Could you check a few things on this model? Use its own coordinates, in mm. Give positions to 0.01 mm unless a question says otherwise; leave off trailing zeros.
1. Imagine slicing it at A-A (y = -387). Count the separate pieces of the cut face and the enclosed holes in it, plus the area to 3 significant figures.
2. For P1, Ø4, axis at y = -136, z = 0, coming from the -X side; P2, Ø3, axis at y = -266, z = -0.5, coming from the +X side; P3, Ø4, axis at x = 1.5, y = -77, coming from the +Z side, each with a flat end and sliding along its axis, tell me the tip position at first contact or that it passes through.
3. I need wall thicknesses on line 1 along Z through (x, y) = (10, -334.5); line 2 along X through (y, z) = (-418.5, -9.5); line 3 along Z through (x, y) = (-11.5, -450). Which ranges of each line are inside material? Lowest first, please.
```python
from build123d import *

# Parameters (mm, degrees)
F0_R     = 3
F0_R_2   = 2.5
F1_DEPTH = 510


with BuildPart() as f1:
    # F0 (on Front) → F1 (new body)
    with BuildSketch(Plane.XZ):
        with BuildLine():
            Line((-4.5, 15), (-14, 15))
            ThreePointArc((-14, 15), (-14.707107, 14.707107), (-15, 14))
            Line((-15, 14), (-15, 4.5))
            ThreePointArc((-15, 4.5), (-14.912132, 4.287868), (-14.7, 4.2))
            Line((-14.7, 4.2), (-14.5, 4.2))
            ThreePointArc((-14.5, 4.2), (-14.146447, 4.053553), (-14, 3.7))
            Line((-14, 3.7), (-14, 3.55))
            ThreePointArc((-14, 3.55), (-13.912132, 3.337868), (-13.7, 3.25))
            Line((-13.7, 3.25), (-12.5, 3.25))
            Line((-12.5, 3.25), (-12.5, 5.25))
            Line((-12.5, 5.25), (-8.004644, 5.25))
            ThreePointArc((-8.004644, 5.25), (-7.629545, 5.176985), (-7.309222, 4.968602))
            Line((-7.309222, 4.968602), (-4.804579, 2.544753))
            ThreePointArc((-4.804579, 2.544753), (-4.579288, 2.216394), (-4.5, 1.826151))
            Line((-4.5, 1.826151), (-4.5, -1.826151))
            ThreePointArc((-4.5, -1.826151), (-4.579288, -2.216394), (-4.804579, -2.544753))
            Line((-4.804579, -2.544753), (-7.309222, -4.968602))
            ThreePointArc((-7.309222, -4.968602), (-7.629545, -5.176985), (-8.004644, -5.25))
            Line((-8.004644, -5.25), (-12.5, -5.25))
            Line((-12.5, -5.25), (-12.5, -3.25))
            Line((-12.5, -3.25), (-13.7, -3.25))
            ThreePointArc((-13.7, -3.25), (-13.912132, -3.337868), (-14, -3.55))
            Line((-14, -3.55), (-14, -3.7))
            ThreePointArc((-14, -3.7), (-14.146447, -4.053553), (-14.5, -4.2))
            Line((-14.5, -4.2), (-14.7, -4.2))
            ThreePointArc((-14.7, -4.2), (-14.912132, -4.287868), (-15, -4.5))
            Line((-15, -4.5), (-15, -14))
            ThreePointArc((-15, -14), (-14.707107, -14.707107), (-14, -15))
            Line((-14, -15), (-4.5, -15))
            ThreePointArc((-4.5, -15), (-4.287868, -14.912132), (-4.2, -14.7))
            Line((-4.2, -14.7), (-4.2, -14.5))
            ThreePointArc((-4.2, -14.5), (-4.053553, -14.146447), (-3.7, -14))
            Line((-3.7, -14), (-3.55, -14))
            ThreePointArc((-3.55, -14), (-3.337868, -13.912132), (-3.25, -13.7))
            Line((-3.25, -13.7), (-3.25, -12.5))
            Line((-3.25, -12.5), (-5.25, -12.5))
            Line((-5.25, -12.5), (-5.25, -8.004644))
            ThreePointArc((-5.25, -8.004644), (-5.176985, -7.629545), (-4.968602, -7.309222))
            Line((-4.968602, -7.309222), (-2.544753, -4.804579))
            ThreePointArc((-2.544753, -4.804579), (-2.216394, -4.579288), (-1.826151, -4.5))
            Line((-1.826151, -4.5), (1.826151, -4.5))
            ThreePointArc((1.826151, -4.5), (2.216394, -4.579288), (2.544753, -4.804579))
            Line((2.544753, -4.804579), (4.968602, -7.309222))
            ThreePointArc((4.968602, -7.309222), (5.176985, -7.629545), (5.25, -8.004644))
            Line((5.25, -8.004644), (5.25, -12.5))
            Line((5.25, -12.5), (3.25, -12.5))
            Line((3.25, -12.5), (3.25, -13.7))
            ThreePointArc((3.25, -13.7), (3.337868, -13.912132), (3.55, -14))
            Line((3.55, -14), (3.7, -14))
            ThreePointArc((3.7, -14), (4.053553, -14.146447), (4.2, -14.5))
            Line((4.2, -14.5), (4.2, -14.7))
            ThreePointArc((4.2, -14.7), (4.287868, -14.912132), (4.5, -15))
            Line((4.5, -15), (14, -15))
            ThreePointArc((14, -15), (14.707107, -14.707107), (15, -14))
            Line((15, -14), (15, -4.5))
            ThreePointArc((15, -4.5), (14.912132, -4.287868), (14.7, -4.2))
            Line((14.7, -4.2), (14.5, -4.2))
            ThreePointArc((14.5, -4.2), (14.146447, -4.053553), (14, -3.7))
            Line((14, -3.7), (14, -3.55))
            ThreePointArc((14, -3.55), (13.912132, -3.337868), (13.7, -3.25))
            Line((13.7, -3.25), (12.5, -3.25))
            Line((12.5, -3.25), (12.5, -5.25))
            Line((12.5, -5.25), (8.004644, -5.25))
            ThreePointArc((8.004644, -5.25), (7.629545, -5.176985), (7.309222, -4.968602))
            Line((7.309222, -4.968602), (4.804579, -2.544753))
            ThreePointArc((4.804579, -2.544753), (4.579288, -2.216394), (4.5, -1.826151))
            Line((4.5, -1.826151), (4.5, 1.826151))
            ThreePointArc((4.5, 1.826151), (4.579288, 2.216394), (4.804579, 2.544753))
            Line((4.804579, 2.544753), (7.309222, 4.968602))
            ThreePointArc((7.309222, 4.968602), (7.629545, 5.176985), (8.004644, 5.25))
            Line((8.004644, 5.25), (12.5, 5.25))
            Line((12.5, 5.25), (12.5, 3.25))
            Line((12.5, 3.25), (13.7, 3.25))
            ThreePointArc((13.7, 3.25), (13.912132, 3.337868), (14, 3.55))
            Line((14, 3.55), (14, 3.7))
            ThreePointArc((14, 3.7), (14.146447, 4.053553), (14.5, 4.2))
            Line((14.5, 4.2), (14.7, 4.2))
            ThreePointArc((14.7, 4.2), (14.912132, 4.287868), (15, 4.5))
            Line((15, 4.5), (15, 14))
            ThreePointArc((15, 14), (14.707107, 14.707107), (14, 15))
            Line((14, 15), (4.5, 15))
            ThreePointArc((4.5, 15), (4.287868, 14.912132), (4.2, 14.7))
            Line((4.2, 14.7), (4.2, 14.5))
            ThreePointArc((4.2, 14.5), (4.053553, 14.146447), (3.7, 14))
            Line((3.7, 14), (3.55, 14))
            ThreePointArc((3.55, 14), (3.337868, 13.912132), (3.25, 13.7))
            Line((3.25, 13.7), (3.25, 12.5))
            Line((3.25, 12.5), (5.25, 12.5))
            Line((5.25, 12.5), (5.25, 8.004644))
            ThreePointArc((5.25, 8.004644), (5.176985, 7.629545), (4.968602, 7.309222))
            Line((4.968602, 7.309222), (2.544753, 4.804579))
            ThreePointArc((2.544753, 4.804579), (2.216394, 4.579288), (1.826151, 4.5))
            Line((1.826151, 4.5), (-1.826151, 4.5))
            ThreePointArc((-1.826151, 4.5), (-2.216394, 4.579288), (-2.544753, 4.804579))
            Line((-2.544753, 4.804579), (-4.968602, 7.309222))
            ThreePointArc((-4.968602, 7.309222), (-5.176985, 7.629545), (-5.25, 8.004644))
            Line((-5.25, 8.004644), (-5.25, 12.5))
            Line((-5.25, 12.5), (-3.25, 12.5))
            Line((-3.25, 12.5), (-3.25, 13.7))
            ThreePointArc((-3.25, 13.7), (-3.337868, 13.912132), (-3.55, 14))
            Line((-3.55, 14), (-3.7, 14))
            ThreePointArc((-3.7, 14), (-4.053553, 14.146447), (-4.2, 14.5))
            Line((-4.2, 14.5), (-4.2, 14.7))
            ThreePointArc((-4.2, 14.7), (-4.287868, 14.912132), (-4.5, 15))
        make_face()
        with Locations((-10, -10)):
            Circle(F0_R, mode=Mode.SUBTRACT)
        with Locations((10, -10)):
            Circle(F0_R, mode=Mode.SUBTRACT)
        with Locations((-10, 10)):
            Circle(F0_R, mode=Mode.SUBTRACT)
        Circle(F0_R_2, mode=Mode.SUBTRACT)
        with Locations((10, 10)):
            Circle(F0_R, mode=Mode.SUBTRACT)
    extrude(amount=F1_DEPTH)


solid = f1.part
```
Derived:
1. separate pieces: 1
1. enclosed holes: 5
1. area: 395 mm2
2. P1: stops at x = -4.52
2. P2: stops at x = 4.52
2. P3: stops at z = 14
3. line 1: z = -15 to -13, -7 to -5.25, 5.25 to 7, 13 to 15
3. line 2: x = -15 to -12.96, -7.04 to -5.25, 5.25 to 7.04, 12.96 to 15
3. line 3: z = -15 to -12.6, -7.4 to -5.25, 5.25 to 7.4, 12.6 to 15
